Input: part model. Units: mm. Frame: model coordinates. Face numbers are marked on the shaded views. A direction names the side the tool comes from. Give positions to 0.01 mm unless a question says otherwise; leave off trailing zeros. Order: outer loops, then holes, each group sorted by start corner. A loop starts at its lowest first (then second) coordinate and runs counter-clockwise, first axis right, second up. Notation, with made-up numbers: (70.5, 56) - (98.5, 56) arc R12 cw to (98.5, 60) - close; hole circle Ø5 at (57, -2.5). An arc over 180 degrees is marked (long way). Answer in a Markdown table with one row per item. Add a question column.
1. Ray query, line 1 (Y direction, x = -21, z = 8.5); line 2 (X direction, y = 19.5, z = 65); line 3 (Z direction, x = 33.5, y = 127.5). Return the intervals inside material, ascending. Write a range as [from, to].
2. Contact query for flat-ended pins moving along their axis: pin 1 (3 mm diameter, centred on y = 93, z = 42.5, fed in from -X); pin 2 (6 mm diameter, centred on x = -10.5, z = -60.5, fed in from +Y); pin 3 (4 mm diameter, centred on x = 38.5, y = 90.5, fed in from +Z); pin 4 (16 mm diameter, centred on x = -20, z = 65, fed in from -Y). Output: stop coordinate, or through.
3. Section query A-A on z = 0. Return loops of the section in (x, y).
4. Section query B-B on y = 385. Return loops of the section in (x, z).
5. Section query C-C on z = 40. Return loops of the section in (x, y), and give its area (3 significant figures).
6. Section query D-D on y = 166. Return loops of the section in (x, z).
7. Access query for the marked faces 1, 2, 3, 4 and 5. Directions: +Z, -Z, +X, -X, +Y, -Y. A direction counts if a zero-diameter tool reaches every point of the face in a straight line with its end or side. Return the directions, or none.
```python
from build123d import *

# Parameters (mm, degrees)
ESQUISSE1_R        = 10
BOSS_EXTRU_1_DEPTH = 25
BOSS_EXTRU_2_DEPTH = 35
BOSS_EXTRU_3_START = -35
ESQUISSE2_4_R      = 50
ESQUISSE2_4_R_2    = 20
BOSS_EXTRU_3_DEPTH = 45


with BuildPart() as part:
    # Esquisse1 → Boss.-Extru.1 (new body)
    with BuildSketch(Plane(origin=(0, 0, 0), x_dir=(1, 0, 0), z_dir=(0, 1, 0))):
        with BuildLine():
            Line((45, -90), (-20, -90))
            ThreePointArc((-20, -90), (-37.67766953, -82.67766953), (-45, -65))
            Line((-45, -65), (-45, 65))
            ThreePointArc((-45, 65), (-37.67766953, 82.67766953), (-20, 90))
            Line((-20, 90), (45, 90))
            Line((45, 90), (45, -90))
        make_face()
        with Locations(Location((-20, 65, 0), (0, 0, 270))):
            Circle(ESQUISSE1_R, mode=Mode.SUBTRACT)
        with Locations(Location((-20, -65, 0), (0, 0, 270))):
            Circle(ESQUISSE1_R, mode=Mode.SUBTRACT)
    extrude(amount=BOSS_EXTRU_1_DEPTH)

    # Esquisse2 → Boss.-Extru.2 (add)
    with BuildSketch(Plane(origin=(45, 0, 0), x_dir=(0, 0, -1), z_dir=(1, 0, 0))):
        with BuildLine():
            Line((-75, 25), (0, 25))
            Line((0, 25), (0, 350))
            ThreePointArc((0, 350), (-35.355339059, 364.644660941), (-50, 400))
            Line((-50, 400), (-50, 50))
            ThreePointArc((-50, 50), (-57.32233047, 32.32233047), (-75, 25))
        make_face()
        with BuildLine():
            Line((0, 350), (0, 25))
            Line((0, 25), (75, 25))
            ThreePointArc((75, 25), (57.32233047, 32.32233047), (50, 50))
            Line((50, 50), (50, 400))
            ThreePointArc((50, 400), (35.355339059, 364.644660941), (0, 350))
        make_face()
    extrude(amount=-BOSS_EXTRU_2_DEPTH)

    # Esquisse2<4> → Boss.-Extru.3 (add)
    with BuildSketch(Plane(origin=(45, 0, 0), x_dir=(0, 0, -1), z_dir=(1, 0, 0)).offset(BOSS_EXTRU_3_START)):
        with Locations((0, 400)):
            Circle(ESQUISSE2_4_R)
        with Locations((0, 400)):
            Circle(ESQUISSE2_4_R_2, mode=Mode.SUBTRACT)
    extrude(amount=BOSS_EXTRU_3_DEPTH)


solid = part.part
```
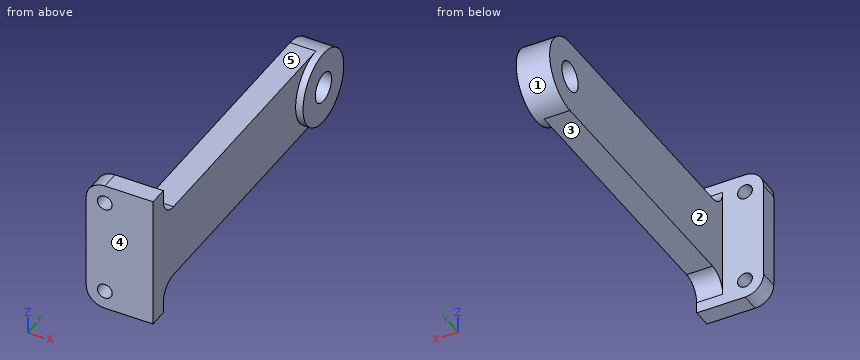
Answer:
| question | item | result |
|---|---|---|
| 1 | line 1 | y = [0, 25] |
| 1 | line 2 | x = [-45, -30], [-10, 45] |
| 1 | line 3 | z = [-50, 50] |
| 2 | pin 1 | stops at x = 10 |
| 2 | pin 2 | stops at y = 25 |
| 2 | pin 3 | stops at z = 50 |
| 2 | pin 4 | passes through |
| 3 | outline | (-45, 0) - (45, 0) - (45, 350) - (55, 350) - (55, 380) - (10, 380) - (10, 25) - (-45, 25) - close; (10, 420) - (55, 420) - (55, 450) - (10, 450) - close |
| 4 | outline | (10, -50) - (45, -50) - (45, -47.7) - (55, -47.7) - (55, -13.23) - (10, -13.23) - close; (10, 13.23) - (55, 13.23) - (55, 47.7) - (45, 47.7) - (45, 50) - (10, 50) - close |
| 5 | outline | (-45, 0) - (45, 0) - (45, 370) - (55, 370) - (55, 430) - (10, 430) - (10, 25) - (-45, 25) - close |
| 5 | area | 17,000 mm² |
| 6 | outline | (10, -50) - (45, -50) - (45, 50) - (10, 50) - close |
| 7 | face 1 | +X |
| 7 | face 2 | +Z, -Z, -X, +Y |
| 7 | face 3 | -Z, +X, -X, +Y |
| 7 | face 4 | +Z, -Z, +X, -X, -Y |
| 7 | face 5 | +Z, +X, -X, +Y |
